The model under review builds one solid part; all positions refer to its coordinate system, in mm. Coordinates: 2 decimals unless noted, no trailing zeros. Loops run counter-clockwise (first coordinate to the right, second up) from the corner with the lowest first, then second, coordinate; pieces in that order, holes last. Notation, with made-up numbers: M 25.5,59 L 60.5,59 A24 ccw 60.5,90 Z; hole C 54,-10 d4. An arc over 180 degrees is marked long. Return JSON: item names as keys, results as strings.
Autodesk Inventor part; units mm, degrees
ref_plane "YZ Plane" through (0, 0, 0) normal (1, 0, 0) x (0, 1, 0)
ref_plane "XZ Plane" through (0, 0, 0) normal (0, 1, 0) x (-1, 0, 0)
ref_plane "XY Plane" through (0, 0, 0) normal (0, 0, 1) x (1, 0, 0)
sketch "Sketch1" plane through (0, 0, 0) normal (0, 0, 1) x (1, 0, 0)
  line L0 (0, 4) -> (1, 4) construction
  line L1 (15, 4) -> (16, 5)
  line L2 (16, 5) -> (54, 5)
  line L3 (0, 4) -> (0, 3) construction
  line L4 (54, 5) -> (55, 6)
  line L5 (55, 6) -> (789, 6)
  line L6 (0, 3) -> (1, 4)
  line L7 (0, 3) -> (0, 0)
  line L8 (1, 4) -> (15, 4)
  line L9 (789, 6) -> (790, 5)
  line L10 (790, 5) -> (790, 4)
  line L11 (790, 4) -> (797, 4)
  line L12 (797, 4) -> (797, 3.8)
  line L13 (797, 3.8) -> (797.9, 3.8)
  line L14 (797.9, 3.8) -> (797.9, 4)
  line L15 (797.9, 4) -> (799, 4)
  line L16 (799, 4) -> (800, 3)
  line L17 (800, 3) -> (800, 0)
  line L18 (0, 0) -> (800, 0)
  point P0 (0, 0)
  point P1 (800, 1.5)
  dimension "d0" = 4
  dimension "d1" = 5
  dimension "d2" = 6
  dimension "d3" = 135
  dimension "d4" = 135
  dimension "d5" = 15
  dimension "d6" = 39
  dimension "d7" = 135
  dimension "d8" = 4
  dimension "d9" = 7
  dimension "d10" = 10
  dimension "d11" = 0.2
  dimension "d12" = 0.9
  dimension "d14" = 135
  dimension "d15" = 800
revolve "Revolution1" add sketch "Sketch1" angle 360 about axis through (0, 0, 0) along (1, 0, 0)
equation "\"SHAFT_LEN\" = 800"
properties part number "SFU1204-800"
1. Add section C-C on x = 87. Give the boundary of the cut face in (y, z).
Check values:
{"outline": "C 0,0 d12"}
2. To check wall thickness, follow line 1 (Z direction, x = 441, y = -1); line 2 (Z direction, x = 423.5, y = 0.75); line 3 (Y direction, x = 674.5, z = -3.25). State the ranges of each line that lie inside material, in increasing order.
Check values:
{"line 1": "-5.92 to 5.92", "line 2": "-5.95 to 5.95", "line 3": "-5.04 to 5.04"}
3. Insertion check: pin 1 Ø3 at (x, y) = (503, -2.5) entering from +Z; pin 2 Ø3 at (x, y) = (215, -2) entering from +Z; pin 3 Ø6 at (x, z) = (394, -4.5) entering from -Y. Each pin has a flat end and moves straight along its axis. Give the tip position at first contact, or say it passes through.
Check values:
{"pin 1": "z = 5.92", "pin 2": "z = 5.98", "pin 3": "y = -5.81"}
